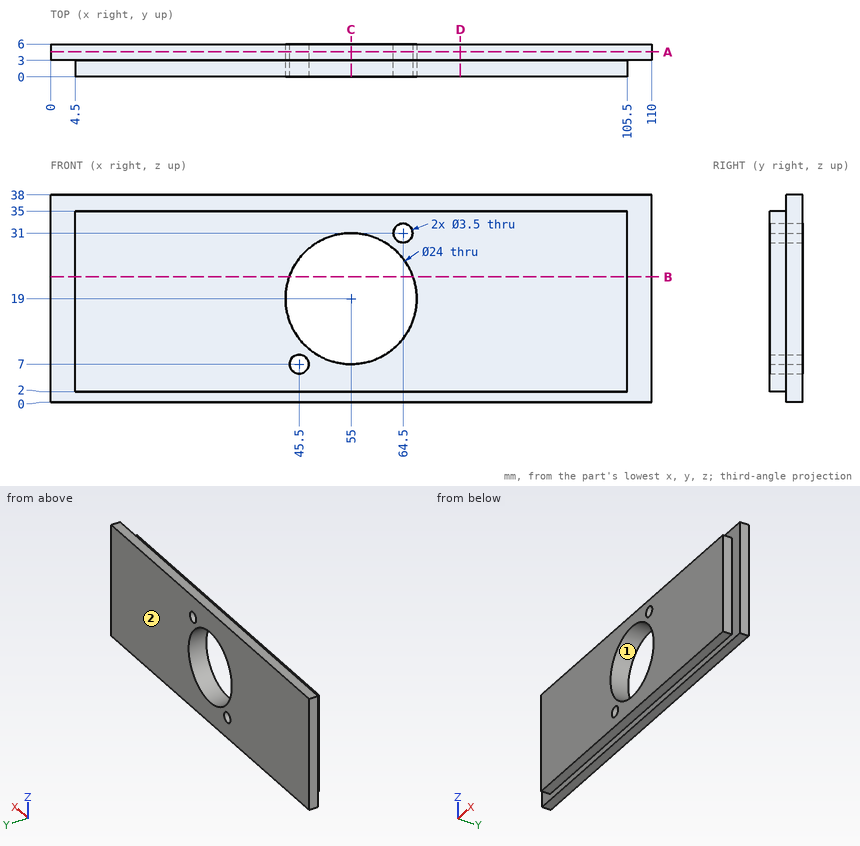
For this review, use the dimensioned drawing (mm, ordinates from the lowest corner) and the shaded views. Coordinates: 2 decimals unless noted, no trailing zeros. Order: outer loops, then holes, each group sorted by start corner. A loop starts at its lowest first (then second) coordinate and runs counter-clockwise, first axis right, second up. Notation, with made-up numbers: (30.5, 19.5) - (51.5, 19.5) arc R20 cw to (51.5, 31.5) - close; hole circle Ø6 at (76, 42.5). An arc over 180 degrees is marked (long way). Answer as a JSON object with one key per item and string values. Group by question number.
1. For probe 1 along X at (y, z) = (3.4, 19); probe 2 along Z at (x, y) = (45.5, 2); probe 3 along Z at (x, y) = (45.5, 3.6), list the stretches that pass through material, from the lowest coordinate up.
2. We need section C-C on x = 55. State the section outline as (y, z) points, then the cut area to 3 significant figures.
3. We need section B-B on z = 23. State the section outline as (x, y) points.
4. We need section A-A on y = 4.55. State the section outline as (x, z) points, then the cut area to 3 significant figures.
5. We need section D-D on x = 75. State the section outline as (y, z) points, then the cut area to 3 significant figures.
6. The part is to be moulded in two halves that separate along Z. For the marked faces 1 and 2, say which applies: pulls with the +Z half, pulls with the -Z half, needs draft (parallel to the pull), parting line crosses it, or undercut.
7. Clearance check with flat-ended pins moving along their axes: P1, Ø2.5, axis at x = 60, y = 1, coming from the -Z side; P2, Ø1.5, axis at x = 43.5, y = 1.5, coming from the +Z side; P3, Ø0.9, axis at y = 2, z = 11.5, coming from the +X side. State where each tip first meets the part, or that it passes through.
Final values:
{
 "1": {"probe 1": "0 to 43, 67 to 110", "probe 2": "2 to 5.25, 8.75 to 11.67, 26.33 to 35", "probe 3": "0 to 5.25, 8.75 to 11.67, 26.33 to 38"},
 "2": {"outline": "(0, 2) - (3, 2) - (3, 0) - (6, 0) - (6, 7) - (0, 7) - close; (0, 31) - (6, 31) - (6, 38) - (3, 38) - (3, 35) - (0, 35) - close", "area": "69.0 mm²"},
 "3": {"outline": "(0, 3) - (4.5, 3) - (4.5, 0) - (43.69, 0) - (43.69, 6) - (0, 6) - close; (66.31, 0) - (105.5, 0) - (105.5, 3) - (110, 3) - (110, 6) - (66.31, 6) - close"},
 "4": {"outline": "(0, 0) - (110, 0) - (110, 38) - (0, 38) - close; hole circle Ø24 at (55, 19); hole circle Ø3.5 at (45.5, 7); hole circle Ø3.5 at (64.5, 31)", "area": "3,710 mm²"},
 "5": {"outline": "(0, 2) - (3, 2) - (3, 0) - (6, 0) - (6, 38) - (3, 38) - (3, 35) - (0, 35) - close", "area": "213 mm²"},
 "6": {"face 1": "undercut", "face 2": "needs draft"},
 "7": {"P1": "z = 2", "P2": "z = 35", "P3": "x = 105.5"}
}
